from build123d import *

# Parameters (mm, degrees)
SKETCH_1_W           = 35
SKETCH_1_H           = 15
EXTRUDE_1_DEPTH      = 3
EXTRUDE_2_DEPTH      = 1
EXTRUDE_2_DEPTH_BACK = 11
SKETCH_3_R           = 1.75
CUT_EXTRUDE_1_DEPTH  = 22.988633427
CUT_EXTRUDE_2_DEPTH  = 5
SKETCH_6_R           = 1.25
EXTRUDE_3_DEPTH      = 4
FILLET_1_R           = 2
SKETCH_7_W           = 1.104079178
SKETCH_7_H           = 3.426452622
SKETCH_7_W_2         = 1.066007483
EXTRUDE_4_DEPTH      = 3


with BuildPart() as part:
    # 草图1 → 凸台-拉伸1 (new body)
    with BuildSketch(Plane(origin=(0, 0, 0), x_dir=(1, 0, 0), z_dir=(0, 1, 0))):
        Rectangle(SKETCH_1_W, SKETCH_1_H)
    extrude(amount=EXTRUDE_1_DEPTH)

    # 草图2 → 凸台-拉伸2 (add, two sides: drawn at the far end of the back side and taken through both)
    with BuildSketch(Plane(origin=(0, 3, 0), x_dir=(1, 0, 0), z_dir=(0, 1, 0)).offset(-EXTRUDE_2_DEPTH_BACK)):
        with BuildLine():
            Line((-3.9, 6.25), (3.9, 6.25))
            ThreePointArc((3.9, 6.25), (10.15, 0), (3.9, -6.25))
            Line((3.9, -6.25), (-3.9, -6.25))
            ThreePointArc((-3.9, -6.25), (-10.15, 0), (-3.9, 6.25))
        make_face()
    extrude(amount=EXTRUDE_2_DEPTH + EXTRUDE_2_DEPTH_BACK)

    # 草图3 → 切除-拉伸1 (cut, through all)
    with BuildSketch(Plane(origin=(0, 3, 0), x_dir=(1, 0, 0), z_dir=(0, 1, 0))):
        with Locations(Location((-14, 0, 0), (0, 0, 270))):
            Circle(SKETCH_3_R)
        with Locations(Location((14, 0, 0), (0, 0, 270))):
            Circle(SKETCH_3_R)
    extrude(amount=-CUT_EXTRUDE_1_DEPTH, mode=Mode.SUBTRACT)

    # 草图5 → 切除-拉伸2 (cut)
    with BuildSketch(Plane(origin=(0, 4, 0), x_dir=(1, 0, 0), z_dir=(0, 1, 0))):
        with BuildLine():
            Line((-1.414213562, 4.25), (-3.9, 4.25))
            ThreePointArc((-3.9, 4.25), (-8.15, 0), (-3.9, -4.25))
            Line((-3.9, -4.25), (-1.414213562, -4.25))
            ThreePointArc((-1.414213562, -4.25), (-1.125538428, -4.15824829), (-0.942809042, -3.916666667))
            ThreePointArc((-0.942809042, -3.916666667), (0, -3.25), (0.942809042, -3.916666667))
            ThreePointArc((0.942809042, -3.916666667), (1.125538428, -4.15824829), (1.414213562, -4.25))
            Line((1.414213562, -4.25), (3.9, -4.25))
            ThreePointArc((3.9, -4.25), (8.15, 0), (3.9, 4.25))
            Line((3.9, 4.25), (1.414213562, 4.25))
            ThreePointArc((1.414213562, 4.25), (1.125538428, 4.15824829), (0.942809042, 3.916666667))
            ThreePointArc((0.942809042, 3.916666667), (0, 3.25), (-0.942809042, 3.916666667))
            ThreePointArc((-0.942809042, 3.916666667), (-1.125538428, 4.15824829), (-1.414213562, 4.25))
        make_face()
    extrude(amount=-CUT_EXTRUDE_2_DEPTH, mode=Mode.SUBTRACT)

    # 草图6 → 凸台-拉伸3 (add)
    with BuildSketch(Plane(origin=(0, -1, 0), x_dir=(1, 0, 0), z_dir=(0, 1, 0))):
        with Locations(Location((-3.9, 0, 0), (0, 0, 270))):
            Circle(SKETCH_6_R)
        with Locations(Location((3.9, 0, 0), (0, 0, 270))):
            Circle(SKETCH_6_R)
    extrude(amount=EXTRUDE_3_DEPTH)

    # 圆角1
    fillet_1_edges = [part.edges().sort_by_distance(p)[0] for p in [
        (17.5, 1.5, 7.5),
        (-17.5, 1.5, 7.5),
        (-17.5, 1.5, -7.5),
        (17.5, 1.5, -7.5),
    ]]
    fillet(fillet_1_edges, radius=FILLET_1_R)

    # 草图7 → 凸台-拉伸4 (add)
    with BuildSketch(Plane.XZ.offset(8)):
        with Locations((-4.16885069, 0.171322631)):
            Rectangle(SKETCH_7_W, SKETCH_7_H)
        with Locations((3.769097885, 0.171322631)):
            Rectangle(SKETCH_7_W_2, SKETCH_7_H)
    extrude(amount=EXTRUDE_4_DEPTH)


solid = part.part
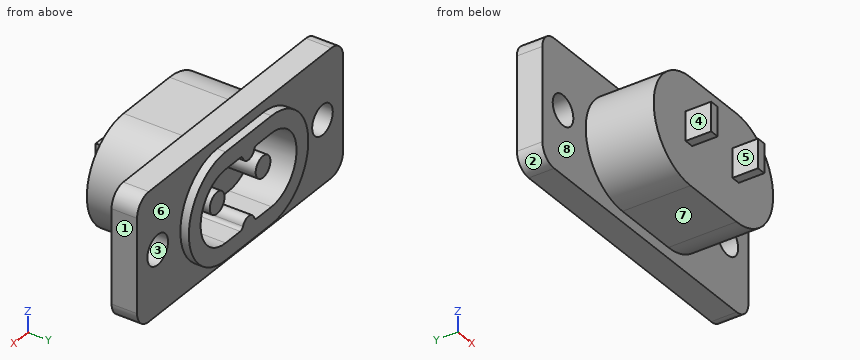
Can you work these out from the model? Positions are in its coordinate system, mm. Face numbers are marked on the shaded views. A direction names the side the tool comes from. Coordinates: 2 decimals unless noted, no trailing zeros. Write each loop counter-clockwise with the first axis right and the second up, starting at its lowest first coordinate (ties: lowest second). Pieces come first, ordered by that corner, then holes.
Q1. Imagine slicing it at A-A, the plane y = 1.5. List the corners of the cut face in (x, z) for me.
Results found:
outline: (-17.5, -5.5) arc R2 ccw to (-15.5, -7.5) - (15.5, -7.5) arc R2 ccw to (17.5, -5.5) - (17.5, 5.5) arc R2 ccw to (15.5, 7.5) - (-15.5, 7.5) arc R2 ccw to (-17.5, 5.5) - close; circle Ø2.5 at (-3.9, 0); circle Ø2.5 at (3.9, 0); hole circle Ø3.5 at (-14, 0); hole (-3.9, -4.25) - (-1.41, -4.25) arc R0.5 ccw to (-0.94, -3.92) arc R1 cw to (0.94, -3.92) arc R0.5 ccw to (1.41, -4.25) - (3.9, -4.25) arc R4.25 ccw to (3.9, 4.25) - (1.41, 4.25) arc R0.5 ccw to (0.94, 3.92) arc R1 cw to (-0.94, 3.92) arc R0.5 ccw to (-1.41, 4.25) - (-3.9, 4.25) arc R4.25 ccw to start; hole circle Ø3.5 at (14, 0)
Q2. If we mould it in two halves opening along Z, with no side actions, what happens to the marked faces 1, 2 and 3? For each: +Z half, -Z half, draft (parallel to the pull), parting line (faces both ways), or undercut.
Results found:
face 1: draft
face 2: -Z half
face 3: undercut
Q3. Please list where these lines run through material, in increasing order: L1, parallel to X at y = 1.45, z = 0; L2, parallel to X at y = 1.25, z = -1; L3, parallel to Z at x = -2, y = -0.5.
Results found:
L1: x = -17.5 to -15.75, -12.25 to -8.15, -5.15 to -2.65, 2.65 to 5.15, 8.15 to 12.25, 15.75 to 17.5
L2: x = -17.5 to -15.44, -12.56 to -8.03, -4.65 to -3.15, 3.15 to 4.65, 8.03 to 12.56, 15.44 to 17.5
L3: z = -6.25 to -4.25, 4.25 to 6.25
Q4. Which directions (+Z, -Z, +X, -X, +Y, -Y) give clear straight access to the entire face, cutting with the end or side of a thin tool? Please do the marked faces 4, 5, 6, 7 and 8.
Results found:
face 4: +Z, -Z, -X, -Y
face 5: +Z, -Z, -Y
face 6: +Y
face 7: -Z, +X, -X, -Y
face 8: -Y
Q5. For P1, Ø1, axis at x = -11, z = 1, coming from the -Y side; P2, Ø0.5, axis at x = 4, y = -9, coming from the -Z side; P3, Ø7.5, axis at x = 4.5, z = -1, coming from the -Y side; P4, Ø1, axis at x = -10.5, z = 3, coming from the +Y side, each with a flat end and sliding along its axis, tell me the tip position at first contact or that it passes through.
Results found:
P1: stops at y = 0
P2: stops at z = -1.54
P3: stops at y = -11
P4: stops at y = 3
Q6. Imagine slicing it at C-C, the plane y = -9.25. List the corners of the cut face in (x, z) for me.
Results found:
outline: (-4.72, -1.54) - (-3.62, -1.54) - (-3.62, 1.88) - (-4.72, 1.88) - close; (3.24, -1.54) - (4.3, -1.54) - (4.3, 1.88) - (3.24, 1.88) - close
Q7. Imagine slicing it at B-B, the plane x = 0. List the corners of the cut face in (y, z) for me.
Results found:
outline: (-8, -6.25) - (0, -6.25) - (0, -7.5) - (3, -7.5) - (3, -6.25) - (4, -6.25) - (4, -3.25) - (-1, -3.25) - (-1, 3.25) - (4, 3.25) - (4, 6.25) - (3, 6.25) - (3, 7.5) - (0, 7.5) - (0, 6.25) - (-8, 6.25) - close
Q8. Imagine slicing it at D-D, the plane z = 5. List the corners of the cut face in (x, y) for me.
Results found:
outline: (-17.5, 0) - (-7.65, 0) - (-7.65, -8) - (7.65, -8) - (7.65, 0) - (17.5, 0) - (17.5, 3) - (7.65, 3) - (7.65, 4) - (-7.65, 4) - (-7.65, 3) - (-17.5, 3) - close
